Verification items for the finished model (mm, model axes). A direction names the side the tool comes from. Coordinates: 2 decimals unless noted, no trailing zeros. Order: outer loops, then holes, each group sorted by start corner. A loop starts at its lowest first (then second) coordinate and runs counter-clockwise, first axis right, second up. Notation, with made-up numbers: (19, 31) -> (32, 31) arc R29 ccw to (32, 56) -> close; hole circle Ø2 at (-21.5, -24). An arc over 180 degrees is marked (long way). Use CSV: the item, a comma, the result in double quotes. Start each with the question number.
1) Sectioned sample at C-C on y = 12.5. Record the boundary of the cut face in (x, z), then the cut area to 3 significant figures.
2) Sectioned sample at A-A on x = 0. Record the boundary of the cut face in (y, z).
3) Scan lines: line 1 along Y through (x, z) = (-34, -14); line 2 along X through (y, z) = (16.5, 5); line 3 along X through (y, z) = (4, -15.5). Record each from-to range of solid material in increasing order.
4) Sectioned sample at B-B on z = 0. Record the boundary of the cut face in (x, y).
5) Sectioned sample at D-D on x = -22.5. Record the boundary of the cut face in (y, z), then the cut area to 3 significant figures.
6) Tool access check on faces 1 (the cylindrical face through (-8.486, 9.86, -16.315)), 2 (the flat face through (0, 20, 0)). Record the directions out of +Z, -Z, +X, -X, +Y, -Y that give a thin tool (end or side, any length) a straight path to the whole face; none if there is none.
from build123d import *

# Parameters (mm, degrees)
SKIZZE1_W                          = 75
SKIZZE1_H                          = 40
AUFSATZ_LINEAR_AUSTRAGEN1_DEPTH    = 40
SKIZZE2_R                          = 18.39
AUFSATZ_LINEAR_AUSTRAGEN2_DEPTH    = 20
K_RPER_VERSCHIEBEN_KOPIEREN1_ANGLE = 180
K_RPER_VERSCHIEBEN_KOPIEREN2_ANGLE = 90
K_RPER_VERSCHIEBEN_KOPIEREN3_ANGLE = 180


with BuildPart() as part:
    # Skizze1 → Aufsatz-Linear austragen1 (new body)
    with BuildSketch(Plane.XY):
        Rectangle(SKIZZE1_W, SKIZZE1_H)
    extrude(amount=AUFSATZ_LINEAR_AUSTRAGEN1_DEPTH)

    # Skizze2 → Aufsatz-Linear austragen2 (add)
    with BuildSketch(Plane(origin=(0, 0, 0), x_dir=(-1, 0, 0), z_dir=(0, 0, -1))):
        Circle(SKIZZE2_R)
    extrude(amount=AUFSATZ_LINEAR_AUSTRAGEN2_DEPTH)


with BuildPart() as part_1:
    # Körper-Verschieben/Kopieren1: moved
    add(part.part.rotate(Axis((0, 0, 10), (1, 0, 0)), K_RPER_VERSCHIEBEN_KOPIEREN1_ANGLE))


with BuildPart() as part_2:
    # Körper-Verschieben/Kopieren2: moved
    add(part_1.part.rotate(Axis((0, 0, 10), (1, 0, 0)), K_RPER_VERSCHIEBEN_KOPIEREN2_ANGLE))


with BuildPart() as part_3:
    # Körper-Verschieben/Kopieren3: moved
    add(part_2.part.rotate(Axis((0, 0, 10), (1, 0, 0)), K_RPER_VERSCHIEBEN_KOPIEREN3_ANGLE))


with BuildPart() as part_4:
    # Körper-Verschieben/Kopieren4: moved
    add(part_3.part.moved(Location((0, -10, 0))))


with BuildPart() as part_5:
    # Körper-Verschieben/Kopieren5: moved
    add(part_4.part.moved(Location((0, 0, -10))))


solid = part_5.part
Answers follow:
1,outline,"circle Ø36.78 at (0, 0)"
1,area,"1,060 mm²"
2,outline,"(-40, -20) -> (0, -20) -> (0, -18.39) -> (20, -18.39) -> (20, 18.39) -> (0, 18.39) -> (0, 20) -> (-40, 20) -> close"
3,line 1,"y = -40 to 0"
3,line 2,"x = -17.7 to 17.7"
3,line 3,"x = -9.9 to 9.9"
4,outline,"(-37.5, -40) -> (37.5, -40) -> (37.5, 0) -> (18.39, 0) -> (18.39, 20) -> (-18.39, 20) -> (-18.39, 0) -> (-37.5, 0) -> close"
5,outline,"(-40, -20) -> (0, -20) -> (0, 20) -> (-40, 20) -> close"
5,area,"1,600 mm²"
6,face 1,"+Y"
6,face 2,"+Z, -Z, +X, -X, +Y"
